```python
from build123d import *

# Parameters (mm, degrees)
F0_R     = 7
F0_R_2   = 1.5
F1_DEPTH = 3
F2_R     = 1.551902
F3_DEPTH = 1.5
F4_W     = 0.3
F4_H     = 6
F5_DEPTH = 6
F6_R     = 2


with BuildPart() as f1:
    # F0 (on Top) → F1 (new body)
    with BuildSketch(Plane.XY):
        Circle(F0_R)
        Circle(F0_R_2, mode=Mode.SUBTRACT)
    extrude(amount=F1_DEPTH)

    # F2 (on face) → F3 (join)
    with BuildSketch(Plane(origin=(0, 0, 0), x_dir=(1, 0, 0), z_dir=(0, 0, -1))):
        Circle(F2_R)
    extrude(amount=-F3_DEPTH)

    # F4 (on face) → F5 (join)
    with BuildSketch(Plane(origin=(0, 0, 0), x_dir=(1, 0, 0), z_dir=(0, 0, -1))):
        with Locations((-3.15, 0)):
            Rectangle(F4_W, F4_H)
        with Locations((3.15, 0)):
            Rectangle(F4_W, F4_H)
    extrude(amount=F5_DEPTH)

    # F6
    f6_edges = [f1.edges().sort_by_distance(p)[0] for p in [
        (-3.15, -3, -6),
        (-3.15, 3, -6),
        (3.15, 3, -6),
        (3.15, -3, -6),
    ]]
    fillet(f6_edges, radius=F6_R)


solid = f1.part
```
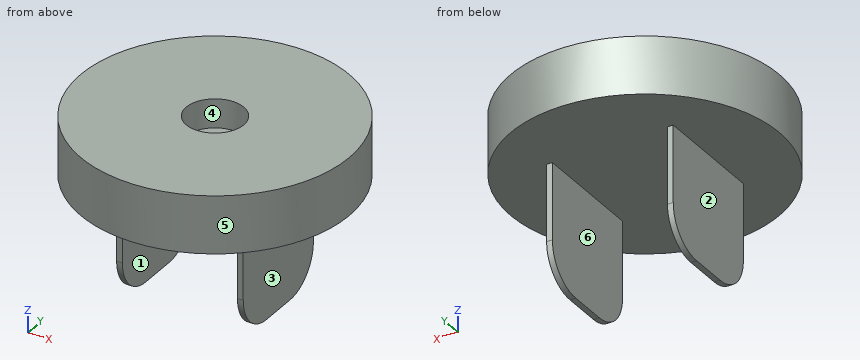
Can you work these out from the model? Positions are in its coordinate system, mm. Face numbers are marked on the shaded views. A direction names the side the tool comes from. Coordinates: 2 decimals unless noted, no trailing zeros. Loops run counter-clockwise (first coordinate to the right, second up) from the corner with the lowest first, then second, coordinate; pieces in that order, holes last. Notation, with made-up numbers: (71, -2.75) - (125, -2.75) arc R20 cw to (125, 2.25) - close; hole circle Ø1 at (-37.5, -2.5). An arc over 180 degrees is marked (long way). Use a Markdown table: item, result.
Item 1: I want a section at A-A on z = -3.75. Please give me the cut outline in (x, y), and give its area (3 significant figures).
Numbers:
| item | result |
|---|---|
| outline | (-3.3, -3) - (-3, -3) - (-3, 3) - (-3.3, 3) - close; (3, -3) - (3.3, -3) - (3.3, 3) - (3, 3) - close |
| area | 3.60 mm2 |
Item 2: We'd pull the mould along X, two halves only. Please class the marked faces 1, 2 and 3: released by +X, released by -X, zero draft, split by the parting line, or undercut.
Numbers:
| item | result |
|---|---|
| face 1 | undercut |
| face 2 | released by -X |
| face 3 | released by +X |
Item 3: If I drill on probe 1 along Y at (x, z) = (0, 2.05); probe 2 along X at (y, z) = (2.75, -4.25); probe 3 along Z at (x, y) = (5.25, 0.75), over which ranges is the centre line in solid material (lowest first)? Write a range as from..to.
Numbers:
| item | result |
|---|---|
| probe 1 | y = -7..-1.5, 1.5..7 |
| probe 2 | x = -3.3..-3, 3..3.3 |
| probe 3 | z = 0..3 |
Item 4: I want a section at D-D on z = 0.25. Please give me the cut outline in (x, y), and give its area (3 significant figures).
Numbers:
| item | result |
|---|---|
| outline | circle Ø14 at (0, 0) |
| area | 154 mm2 |
Item 5: I want a section at C-C on x = 0. Please give me the cut outline in (y, z).
Numbers:
| item | result |
|---|---|
| outline | (-7, 0) - (7, 0) - (7, 3) - (1.5, 3) - (1.5, 1.5) - (-1.5, 1.5) - (-1.5, 3) - (-7, 3) - close |
Item 6: For the marked faces 4, 5 and 6, which set-ups out of +Z, -Z, +X, -X, +Y, -Y let a thin tool reach every point of the face, with its end or its side?
Numbers:
| item | result |
|---|---|
| face 4 | +Z |
| face 5 | +Z, -Z |
| face 6 | -Z, +Y, -Y |
Item 7: Will these pins go through, and if not, where does the flat tip stop? pin 1 (2 mm diameter, centred on x = 1.5, y = -5, fed in from -Z); pin 2 (3 mm diameter, centred on y = -0.5, z = -3.5, fed in from +X); pin 3 (0.9 mm diameter, centred on x = 0, y = 0, fed in from +Z).
Numbers:
| item | result |
|---|---|
| pin 1 | stops at z = 0 |
| pin 2 | stops at x = 3.3 |
| pin 3 | stops at z = 1.5 |
Item 8: I want a section at B-B on y = 0. Please give me the cut outline in (x, z), and give its area (3 significant figures).
Numbers:
| item | result |
|---|---|
| outline | (-7, 0) - (-3.3, 0) - (-3.3, -6) - (-3, -6) - (-3, 0) - (3, 0) - (3, -6) - (3.3, -6) - (3.3, 0) - (7, 0) - (7, 3) - (1.5, 3) - (1.5, 1.5) - (-1.5, 1.5) - (-1.5, 3) - (-7, 3) - close |
| area | 41.1 mm2 |
